from build123d import *

# Parameters (mm, degrees)
BOSS_EXTRUDE1_DEPTH = 14
SKETCH2_R           = 10
BOSS_EXTRUDE2_DEPTH = 160
DOME1_FACE_RADIUS   = 10
DOME1_HEIGHT        = 3


with BuildPart() as part:
    # Sketch1 → Boss-Extrude1 (new body)
    with BuildSketch(Plane(origin=(0, 0, 0), x_dir=(0, 0, -1), z_dir=(1, 0, 0))):
        Polygon((19.629909152, 0.677446241), (9.814954576, 17.677446241), (-9.814954576, 17.677446241), (-19.629909152, 0.677446241), (-9.814954576, -16.322553759), (9.814954576, -16.322553759), align=None)
    extrude(amount=-BOSS_EXTRUDE1_DEPTH)

    # Sketch2 → Boss-Extrude2 (add)
    with BuildSketch(Plane.ZY.offset(14)):
        with Locations((0.23707655, 0.179585486)):
            Circle(SKETCH2_R)
    extrude(amount=BOSS_EXTRUDE2_DEPTH)

    # Dome1: a dome of height H over a round flat face of radius A is a cap of a sphere of radius (A * A + H * H) / (2 * H)
    dome1_r = (DOME1_FACE_RADIUS * DOME1_FACE_RADIUS + DOME1_HEIGHT * DOME1_HEIGHT) / (2 * DOME1_HEIGHT)
    dome1_base = Plane((-174, 0.179585486, 0.23707655), z_dir=(-1, 0, 0))
    with Locations(dome1_base.offset(DOME1_HEIGHT - dome1_r)):
        dome1_ball = Sphere(dome1_r, mode=Mode.PRIVATE)
    add(split(dome1_ball, bisect_by=dome1_base, keep=Keep.TOP, mode=Mode.PRIVATE))

    # Sketch4 → Cut-Revolve4 (revolve, cut)
    with BuildSketch(Plane(origin=(0, 0, 0), x_dir=(1, 0, 0), z_dir=(0, 1, 0))):
        Polygon((0, 18.463333515), (-1.632693956, 21.873968697), (3.881125963, 21.268551199), (2.875714826, 18.463333515), align=None)
    revolve(axis=Axis((0, 0, 0), (1, 0, 0)), mode=Mode.SUBTRACT)


solid = part.part
Geometry: final body of the model. Coordinates: model frame, mm. A direction names the side the tool comes from. Give positions to 0.01 mm unless a question says otherwise; leave off trailing zeros. Loops run counter-clockwise (first coordinate to the right, second up) from the corner with the lowest first, then second, coordinate; pieces in that order, holes last. Notation, with made-up numbers: (37.5, 70.25) - (67.5, 70.25) arc R25 ccw to (67.5, 94.25) - close; hole circle Ø2 at (-33, -38.75). An arc over 180 degrees is marked (long way). Answer as CSV lines item,"result". Start each with the question number.
1. Section C-C, the plane x = -62. Return loops of the section in (y, z).
2. Pin query (flat end, axial travel): P1, Ø1.5, axis at x = -146, z = -8.5, coming from the -Y side; P2, Ø12, axis at x = -107.5, z = 9.5, coming from the -Y side; P3, Ø12, axis at x = -115.5, y = 7, coming from the +Z side. Return the tip coordinate at first contact, or that it passes through.
3. Section B-B, the plane z = 3.5. Return loops of the section in (x, y), plus the area to 3 significant figures.
4. Reachability of faces 1 (the face through (-92.88, 3.183, 9.775)), 2 (the face through (-7, -16.323, 0)) from +Z, -Z, +X, -X, +Y, -Y: full face, straight path, thin tool, end or side. Return the list, or none.
5. Ray query, L1, parallel to X at y = 5, z = 17; L2, parallel to Y at x = -117, z = 7; L3, parallel to X at y = 15, z = -11. Return the intervals inside material, ascending.
6. Section A-A, the plane y = -5. Return loops of the section in (x, z), plus the area to 3 significant figures.
7. Section D-D, the plane z = -15.5. Return loops of the section in (x, y).
Answers:
1,outline,"circle Ø20 at (0.18, 0.24)"
2,P1,"stops at y = -5.84"
2,P2,"stops at y = -9.27"
2,P3,"stops at z = 10.2"
3,outline,"(-174, -9.27) - (-14, -9.27) - (-14, -16.32) - (0, -16.32) - (0, 17.68) - (-14, 17.68) - (-14, 9.63) - (-174, 9.63) arc R17.87 ccw to start"
3,area,"3,540 mm2"
4,face 1,"-X"
4,face 2,"+Z, -Z, +X, -X, -Y"
5,L1,"x = -14 to 0"
5,L2,"y = -7.19 to 7.55"
5,L3,"x = -14 to -0.07"
6,outline,"(-174, -8.32) - (-14, -8.32) - (-14, -16.35) - (0, -16.35) - (0, 16.35) - (-14, 16.35) - (-14, 8.79) - (-174, 8.79) arc R17.41 ccw to start"
6,area,"3,220 mm2"
7,outline,"(-14, -6.48) - (0, -6.48) - (0, 7.83) - (-14, 7.83) - close"
